Source: CAD feature listing. Evaluate the final solid. Frame: model axes, mm. Face numbers are marked on the shaded views. A direction names the side the tool comes from. Coordinates: 2 decimals unless noted, no trailing zeros. Write each loop counter-clockwise with the first axis right and the second up, starting at its lowest first coordinate (ties: lowest second). Pieces come first, ordered by that corner, then holes. Notation, with made-up numbers: M 6.5,39.25 L 13.5,39.25 A30 ccw 13.5,73.25 Z; hole C 23,36 d6. An arc over 180 degrees is marked long. Write item = value, one per line. Start each with the question number.
1. Pull-direction query (X, two-part tool) for the marked faces 3, 4 and 5; classes: pulls with the +X half, pulls with the -X half, needs draft (parallel to the pull), parting line crosses it, or undercut.
2. Section query C-C (z = 29). Give the number of separate pieces and of enclosed holes in the cut face, then the cut area to 3 significant figures.
3. Line query: line 1 along Y through (x, z) = (-58.75, 14.84) (1 decimal); line 2 along X through (y, z) = (-16, 25) (3 decimals); line 3 along Z through (x, y) = (52, 0). Output: solid intervals per line, ascending.
4. Section query A-A (x = 52.5). Output: boundary loops of the cut face in (y, z) (3 decimals), then the cut area to 3 significant figures.
5. Pin query (flat end, axial travel): pin 1 Ø8 at (x, z) = (-52.5, 41.11) entering from -Y (3 decimals); pin 2 Ø8 at (x, z) = (-36.5, 32) entering from +Y (3 decimals); pin 3 Ø5 at (x, z) = (52.5, 8.89) entering from -Y; pin 4 Ø1.6 at (y, z) = (-3.5, 15.5) entering from +X. Return the tip coordinate at first contact, or that it passes through.
6. Section query B-B (x = 0). Output: boundary loops of the cut face in (y, z) (3 decimals), then the cut area to 3 significant figures.
7. Access query for the marked faces 1 and 2. Directions: +Z, -Z, +X, -X, +Y, -Y. A direction counts if a zero-diameter tool reaches every point of the face in a straight line with its end or side. Return the directions, or none.
```python
from build123d import *

# Parameters (mm, degrees)
SKETCH3_W            = 140
SKETCH3_H            = 42.809999978
BOSS_EXTRUDE1_DEPTH  = 50
SKETCH4_R            = 9
CUT_EXTRUDE1_DEPTH   = 50
LPATTERN1_COUNT      = 2
LPATTERN1_PITCH      = 35
LPATTERN1_COL_COUNT  = 2
LPATTERN1_COL_PITCH  = 35
CUT_EXTRUDE2_DEPTH   = 25
LPATTERN2_COUNT      = 2
LPATTERN2_PITCH      = 35
LPATTERN2_COL_COUNT  = 2
LPATTERN2_COL_PITCH  = 35
SKETCH16_R           = 3
CUT_EXTRUDE3_DEPTH   = 90.932
LPATTERN4_COUNT      = 4
LPATTERN4_PITCH      = 35
LPATTERN4_COUNT_DIR2 = 2
LPATTERN4_PITCH_DIR2 = 32.2199
BOSS_EXTRUDE2_START  = -9
SKETCH18_R           = 9
SKETCH18_R_2         = 6.985
BOSS_EXTRUDE2_DEPTH  = 9
CHAMFER1_SIZE        = 1.27
SKETCH21_R           = 1.5875
CUT_EXTRUDE6_DEPTH   = 14
SKETCH22_R           = 1.5875
CUT_EXTRUDE7_DEPTH   = 14


with BuildPart() as part:
    # Sketch3 → Boss-Extrude1 (new body)
    with BuildSketch(Plane.XY):
        Rectangle(SKETCH3_W, SKETCH3_H)
    extrude(amount=BOSS_EXTRUDE1_DEPTH)

    # Sketch4 → Cut-Extrude1 (cut)
    with BuildSketch(Plane(origin=(0, 21.404999989, 0), x_dir=(1, 0, 0), z_dir=(0, 1, 0))):
        with Locations(Location((0, -25, 0), (0, 0, 270))):
            Circle(SKETCH4_R)
    cut_extrude1 = extrude(amount=-CUT_EXTRUDE1_DEPTH, mode=Mode.SUBTRACT)

    # LPattern1: Cut-Extrude1 ×2
    with Locations(*[(i * LPATTERN1_PITCH, 0, 0) for i in range(1, LPATTERN1_COUNT)]):
        add(cut_extrude1, mode=Mode.SUBTRACT)

    # LPattern1 col: Cut-Extrude1 ×2
    with Locations(*[(-i * LPATTERN1_COL_PITCH, 0, 0) for i in range(1, LPATTERN1_COL_COUNT)]):
        add(cut_extrude1, mode=Mode.SUBTRACT)

    # Sketch5 → Cut-Extrude2 (cut)
    with BuildSketch(Plane(origin=(0, 21.404999989, 0), x_dir=(1, 0, 0), z_dir=(0, 1, 0))):
        with BuildLine():
            Line((-6.599113577, -13.43), (-13.31947071, -25.07))
            ThreePointArc((-13.31947071, -25.07), (-13.31947071, -32.69), (-6.720357133, -36.5))
            Line((-6.720357133, -36.5), (6.720357133, -36.5))
            ThreePointArc((6.720357133, -36.5), (13.31947071, -32.69), (13.31947071, -25.07))
            Line((13.31947071, -25.07), (6.599113577, -13.43))
            ThreePointArc((6.599113577, -13.43), (0, -9.62), (-6.599113577, -13.43))
        make_face()
    cut_extrude2 = extrude(amount=-CUT_EXTRUDE2_DEPTH, mode=Mode.SUBTRACT)

    # LPattern2: Cut-Extrude2 ×2
    with Locations(*[(i * LPATTERN2_PITCH, 0, 0) for i in range(1, LPATTERN2_COUNT)]):
        add(cut_extrude2, mode=Mode.SUBTRACT)

    # LPattern2 col: Cut-Extrude2 ×2
    with Locations(*[(-i * LPATTERN2_COL_PITCH, 0, 0) for i in range(1, LPATTERN2_COL_COUNT)]):
        add(cut_extrude2, mode=Mode.SUBTRACT)

    # Sketch16 → Cut-Extrude3 (cut)
    with BuildSketch(Plane(origin=(0, 21.404999989, 0), x_dir=(1, 0, 0), z_dir=(0, 1, 0))):
        with Locations(Location((-52.5, -8.89, 0), (0, 0, 270))):
            Circle(SKETCH16_R)
    cut_extrude3 = extrude(amount=-CUT_EXTRUDE3_DEPTH, mode=Mode.SUBTRACT)

    # LPattern4: Cut-Extrude3 4 × 2
    with Locations(*[(i * LPATTERN4_PITCH, 0, j * LPATTERN4_PITCH_DIR2) for i in range(LPATTERN4_COUNT) for j in range(LPATTERN4_COUNT_DIR2) if (i, j) != (0, 0)]):
        add(cut_extrude3, mode=Mode.SUBTRACT)

    # Sketch18 → Boss-Extrude2 (add)
    # profile 1 of 3: a face of its own
    with BuildSketch(Plane.XZ.offset(21.404999989).offset(BOSS_EXTRUDE2_START)):
        with Locations(Location((0, 25, 0), (0, 0, 90))):
            Circle(SKETCH18_R)
        with Locations(Location((0, 25, 0), (0, 0, 270))):
            Circle(SKETCH18_R_2, mode=Mode.SUBTRACT)
    # profile 2 of 3: a face of its own
    with BuildSketch(Plane.XZ.offset(21.404999989).offset(BOSS_EXTRUDE2_START)):
        with Locations(Location((-35, 25, 0), (0, 0, 90))):
            Circle(SKETCH18_R)
        with Locations(Location((-35, 25, 0), (0, 0, 270))):
            Circle(SKETCH18_R_2, mode=Mode.SUBTRACT)
    # profile 3 of 3: a face of its own
    with BuildSketch(Plane.XZ.offset(21.404999989).offset(BOSS_EXTRUDE2_START)):
        with Locations(Location((35, 25, 0), (0, 0, 90))):
            Circle(SKETCH18_R)
        with Locations(Location((35, 25, 0), (0, 0, 270))):
            Circle(SKETCH18_R_2, mode=Mode.SUBTRACT)
    extrude(amount=BOSS_EXTRUDE2_DEPTH)

    # Chamfer1
    chamfer1_edges = [part.edges().sort_by_distance(p)[0] for p in [
        (0, 21.404999989, 0),
        (-70, 21.404999989, 25),
        (70, 21.404999989, 25),
        (0, 21.404999989, 50),
    ]]
    chamfer(chamfer1_edges, length=CHAMFER1_SIZE)

    # Sketch21 → Cut-Extrude6 (cut)
    with BuildSketch(Plane(origin=(70, 0, 0), x_dir=(0, 0, -1), z_dir=(1, 0, 0))):
        with Locations((-35.16, 8.855000011)):
            Circle(SKETCH21_R)
        with Locations((-35.16, -3.844999989)):
            Circle(SKETCH21_R)
        with Locations((-14.84, -3.844999989)):
            Circle(SKETCH21_R)
        with Locations((-14.84, 8.855000011)):
            Circle(SKETCH21_R)
    extrude(amount=-CUT_EXTRUDE6_DEPTH, mode=Mode.SUBTRACT)

    # Sketch22 → Cut-Extrude7 (cut)
    with BuildSketch(Plane.ZY.offset(70)):
        with Locations((14.84, 8.821000011)):
            Circle(SKETCH22_R)
        with Locations((14.84, -3.878999989)):
            Circle(SKETCH22_R)
        with Locations((35.16, 8.821000011)):
            Circle(SKETCH22_R)
        with Locations((35.16, -3.878999989)):
            Circle(SKETCH22_R)
    extrude(amount=-CUT_EXTRUDE7_DEPTH, mode=Mode.SUBTRACT)


solid = part.part
```
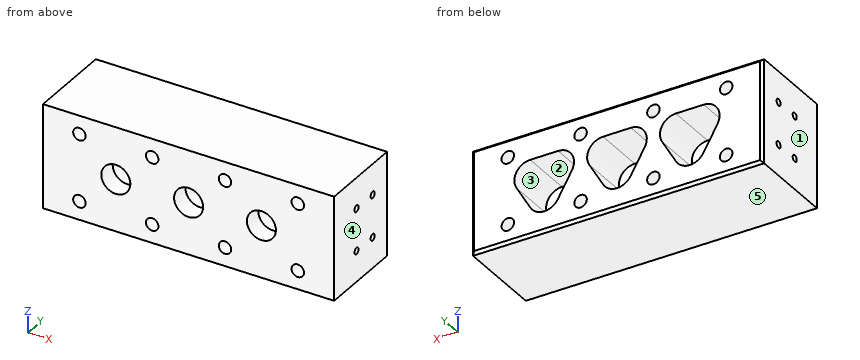
Results are:
q1.face_3 = undercut
q1.face_4 = pulls with the +X half
q1.face_5 = needs draft
q2.separate_pieces = 4
q2.enclosed_holes = 0
q2.area = 3,110 mm^2
q3.line_1 = -21.4 to -5.5, -2.3 to 7.2, 10.4 to 21.4
q3.line_2 = -70 to -41.985, -28.015 to -6.985, 6.985 to 28.015, 41.985 to 70
q3.line_3 = 0 to 5.93, 11.85 to 38.15, 44.07 to 50
q4.outline = M -21.405,0 L 20.135,0 L 21.405,1.27 L 21.405,5.89 L -21.405,5.89 Z; M -21.405,11.89 L 21.405,11.89 L 21.405,38.11 L -21.405,38.11 Z; M -21.405,44.11 L 21.405,44.11 L 21.405,48.73 L 20.135,50 L -21.405,50 Z
q4.area = 1,630 mm^2
q5.pin_1 = -21.405
q5.pin_2 = -3.595
q5.pin_3 = through
q5.pin_4 = 56
q6.outline = M -21.405,0 L 20.135,0 L 21.405,1.27 L 21.405,9.62 L -3.595,9.62 L -3.595,16 L -12.405,16 L -12.405,18.015 L -21.405,18.015 Z; M -21.405,31.985 L -12.405,31.985 L -12.405,34 L -3.595,34 L -3.595,36.5 L 21.405,36.5 L 21.405,48.73 L 20.135,50 L -21.405,50 Z
q6.area = 1,180 mm^2
q7.face_1 = +Z, -Z, -X, +Y, -Y
q7.face_2 = +Y
